```python
from build123d import *

# Parameters (mm, degrees)
EXTRUDE_340_DEPTH = 22.5


with BuildPart() as part:
    # 草图1 → Extrude 340 (new body, symmetric)
    with BuildSketch(Plane.XY):
        Polygon((1.986084926, 3.44), (-1.986084926, 3.44), (-3.972169852, 0), (-1.986084926, -3.44), (1.986084926, -3.44), (3.972169852, 0), align=None)
    extrude(amount=EXTRUDE_340_DEPTH, both=True)

    # 草图3 → 螺纹孔1 (revolve, cut)
    with BuildSketch(Plane(origin=(0, 0, 22.5), x_dir=(0, -1, 0), z_dir=(1, 0, 0))):
        Polygon((0, 0), (0, 14.191420021), (1.65, 13.2), (1.65, 0), align=None)
    hole_wizard_1 = revolve(axis=Axis((0, 0, 28.85), (0, 0, -1)), mode=Mode.SUBTRACT)

    # 镜向1: 螺纹孔1 across plane
    add(hole_wizard_1.mirror(Plane.XY), mode=Mode.SUBTRACT)


solid = part.part
```
Source: CAD feature listing. Evaluate the final solid. Frame: model axes, mm. A direction names the side the tool comes from. Round coordinates to 2 decimals unless told otherwise and drop trailing zeros. Loops run counter-clockwise (first coordinate to the right, second up) from the corner with the lowest first, then second, coordinate; pieces in that order, holes last.
1. Access query for faces 4 (the cylindrical face through (-1.115, 1.216, 15.992)), 5 (the conical face through (0.3, 0.1, -8.5)). Directions: +Z, -Z, +X, -X, +Y, -Y. A direction counts if a zero-diameter tool reaches every point of the face in a straight line with its end or side. Return the directions, or none.
2. Mould query, pull axis X, two halves, no side actions, for faces 1 (the cylindrical face through (-1.115, 1.216, -15.992)), 2 (the flat face through (-2.965, 1.744, 0.315)), 3 (the flat face through (2, 0, 22.5)). Classes: released by +X, released by -X, zero draft, split by the parting line, or undercut.
3. Section query B-B on x = -2.75. Output: boundary loops of the cut face in (y, z), and give its area (3 significant figures).
4. Contact query for flat-ended pins moving along their axis: pin 1 (1.5 mm diameter, centred on y = -0.5, z = 10.5, fed in from +X); pin 2 (2 mm diameter, centred on y = -1.5, z = 17, fed in from +X); pin 3 (4 mm diameter, centred on x = 0, y = 0, fed in from +Z). Output: stop coordinate, or through.
5. Section query A-A on z = 17. Output: boundary loops of the cut face in (x, y), and give its area (3 significant figures).
6. Ray query, L1, parallel to Y at x = 0, z = 17.75; L2, parallel to X at y = 0, z = 16.5; L3, parallel to X at y = -1, z = 20.5. Return the intervals inside material, ascending.
Answers below:
1. face 4: +Z
1. face 5: -Z
2. face 1: undercut
2. face 2: released by -X
2. face 3: zero draft
3. outline: (-2.12, -22.5) - (2.12, -22.5) - (2.12, 22.5) - (-2.12, 22.5) - close
3. area: 191 mm2
4. pin 1: stops at x = 3.97
4. pin 2: stops at x = 3.68
4. pin 3: stops at z = 22.5
5. outline: (-3.97, 0) - (-1.99, -3.44) - (1.99, -3.44) - (3.97, 0) - (1.99, 3.44) - (-1.99, 3.44) - close; hole circle Ø3.3 at (0, 0)
5. area: 32.4 mm2
6. L1: y = -3.44 to -1.65, 1.65 to 3.44
6. L2: x = -3.97 to -1.65, 1.65 to 3.97
6. L3: x = -3.39 to -1.31, 1.31 to 3.39
